Model file for the job. Use its own axes, mm. Give positions to 0.01 mm unless a question says otherwise; leave off trailing zeros. Loops run counter-clockwise (first coordinate to the right, second up) from the corner with the lowest first, then second, coordinate; pieces in that order, holes last. Notation, with made-up numbers: M 66.25,68 L 86.25,68 A29 cw 86.25,98 Z; hole C -22,42.25 d11. An arc over 180 degrees is marked long. Answer in a Markdown table with one row per item.
```python
from build123d import *

# Parameters (mm, degrees)
SKETCH1_R           = 2.875
SKETCH1_R_2         = 7
BOSS_EXTRUDE1_DEPTH = 24.5875
SKETCH4_W           = 66.272407177
SKETCH4_H           = 27.800260981
CUT_EXTRUDE2_DEPTH  = 20
FILLET3_R           = 10
FILLET4_R           = 10
BOSS_EXTRUDE3_START = -1.5875
BOSS_EXTRUDE3_DEPTH = 1.5875
SKETCH7_R           = 7
CUT_EXTRUDE3_DEPTH  = 1.5875
CUT_EXTRUDE4_START  = -10
SKETCH8_R           = 3
SKETCH8_R_2         = 18.9
SKETCH8_R_3         = 2.875
SKETCH8_R_4         = 7
CUT_EXTRUDE4_DEPTH  = 10
SKETCH9_W           = 229.1070397
SKETCH9_H           = 361.266964835
SKETCH9_R           = 1.388229101
SKETCH9_R_2         = 1.483383261
SKETCH9_R_3         = 1.314910669
SKETCH9_R_4         = 1.248623853
SKETCH9_R_5         = 1.255629307
SKETCH9_R_6         = 1.53911217
CUT_EXTRUDE5_DEPTH  = 13
SKETCH10_W          = 29.988446547
SKETCH10_H          = 5
SKETCH10_H_2        = 5.75
CUT_EXTRUDE6_DEPTH  = 22
SKETCH11_R          = 5.236653548
CUT_EXTRUDE7_DEPTH  = 10
BOSS_EXTRUDE4_START = -1.59
BOSS_EXTRUDE4_DEPTH = 1.59
SKETCH13_R          = 7
CUT_EXTRUDE8_DEPTH  = 41
SKETCH14_W          = 61.491848917
SKETCH14_H          = 35.587491391
CUT_EXTRUDE9_DEPTH  = 20
FILLET5_R           = 10
SKETCH16_W          = 163.723031551
SKETCH16_H          = 22.872070304
CUT_EXTRUDE11_DEPTH = 35
FILLET6_R           = 10
SKETCH17_R          = 1.53911217
SKETCH17_R_2        = 1.255629307
SKETCH17_R_3        = 1.3
SKETCH17_R_4        = 1.314910669
SKETCH17_R_5        = 1.388229101
SKETCH17_R_6        = 1.5
CUT_EXTRUDE12_DEPTH = 42
CUT_EXTRUDE13_START = -30
SKETCH18_R          = 18.9
CUT_EXTRUDE13_DEPTH = 30


with BuildPart() as part:
    # Sketch1 → Boss-Extrude1 (new body)
    with BuildSketch(Plane(origin=(0, 0, 0), x_dir=(1, 0, 0), z_dir=(0, 1, 0))):
        with BuildLine():
            Line((42.32729629, 228.6), (10.454309325, 228.6))
            Line((10.454309325, 228.6), (0, 135.362739137))
            Line((0, 135.362739137), (0, 0))
            Line((0, 0), (24.327009544, 0))
            Line((24.327009544, 0), (50.8, 0))
            Line((50.8, 0), (50.8, 64.87909603))
            Line((50.8, 64.87909603), (50.8, 87.423477361))
            Line((50.8, 87.423477361), (50.8, 98.200996728))
            ThreePointArc((50.8, 98.200996728), (50.4, 101.000996728), (50.8, 103.800996728))
            Line((50.8, 103.800996728), (50.8, 104.488200565))
            Line((50.8, 104.488200565), (50.8, 120.619222808))
            Line((50.8, 120.619222808), (50.8, 135.362739137))
            Line((50.8, 135.362739137), (42.32729629, 228.6))
        make_face()
        with Locations(Location((24.101759227, 108.78493524, 0), (0, 0, 270))):
            Circle(SKETCH1_R, mode=Mode.SUBTRACT)
        with Locations(Location((29.504213454, 189.557234372, 0), (0, 0, 270))):
            Circle(SKETCH1_R_2, mode=Mode.SUBTRACT)
    extrude(amount=BOSS_EXTRUDE1_DEPTH)

    # Sketch4 → Cut-Extrude2 (cut)
    with BuildSketch(Plane(origin=(0, 0, -228.6), x_dir=(-1, 0, 0), z_dir=(0, 0, -1))):
        with Locations((-28.174690156, -1.980940155)):
            Rectangle(SKETCH4_W, SKETCH4_H)
    extrude(amount=-CUT_EXTRUDE2_DEPTH, mode=Mode.SUBTRACT)

    # Fillet3
    fillet3_edges = [part.edges().sort_by_distance(p)[0] for p in [
        (44.144746445, 5.959595168, -208.6),
    ]]
    fillet(fillet3_edges, radius=FILLET3_R)

    # Fillet4
    fillet4_edges = [part.edges().sort_by_distance(p)[0] for p in [
        (50.8, 12.29375, 0),
        (0, 12.29375, 0),
        (8.211791854, 5.959595168, -208.6),
    ]]
    fillet(fillet4_edges, radius=FILLET4_R)

    # Sketch6 → Boss-Extrude3 (add)
    with BuildSketch(Plane(origin=(0, 24.5875, 0), x_dir=(1, 0, 0), z_dir=(0, 1, 0)).offset(BOSS_EXTRUDE3_START)):
        with BuildLine():
            Line((50.8, 135.362739137), (50.8, 103.800996728))
            ThreePointArc((50.8, 103.800996728), (50.4, 101.000996728), (50.8, 98.200996728))
            Line((50.8, 98.200996728), (50.8, 61.124243317))
            Line((50.8, 61.124243317), (69.258211507, 96.360728536))
            ThreePointArc((69.258211507, 96.360728536), (70.393157133, 101.370875786), (68.890940865, 106.283413148))
            Line((68.890940865, 106.283413148), (50.8, 135.362739137))
        make_face()
    extrude(amount=BOSS_EXTRUDE3_DEPTH)

    # Sketch7 → Cut-Extrude3 (cut)
    with BuildSketch(Plane(origin=(0, 24.5875, 0), x_dir=(1, 0, 0), z_dir=(0, 1, 0))):
        with Locations(Location((60.4, 101.000996728, 0), (0, 0, 270))):
            Circle(SKETCH7_R)
    extrude(amount=-CUT_EXTRUDE3_DEPTH, mode=Mode.SUBTRACT)

    # Sketch8 → Cut-Extrude4 (cut)
    with BuildSketch(Plane(origin=(0, 24.5875, 0), x_dir=(1, 0, 0), z_dir=(0, 1, 0)).offset(CUT_EXTRUDE4_START)):
        with BuildLine():
            Line((10.454309325, 228.6), (0, 135.362739137))
            Line((0, 135.362739137), (0, 10))
            ThreePointArc((0, 10), (2.928932188, 2.928932188), (10, 0))
            Line((10, 0), (40.8, 0))
            ThreePointArc((40.8, 0), (47.871067812, 2.928932188), (50.8, 10))
            Line((50.8, 10), (50.8, 61.124243317))
            Line((50.8, 61.124243317), (69.258211507, 96.360728536))
            ThreePointArc((69.258211507, 96.360728536), (70.393157133, 101.370875786), (68.890940865, 106.283413148))
            Line((68.890940865, 106.283413148), (50.8, 135.362739137))
            Line((50.8, 135.362739137), (42.32729629, 228.6))
            Line((42.32729629, 228.6), (10.454309325, 228.6))
        make_face()
        with Locations(Location((9.492033273, 118.909935242, 0), (0, 0, 270))):
            Circle(SKETCH8_R, mode=Mode.SUBTRACT)
        with Locations(Location((24.583834565, 64.593886665, 0), (0, 0, 270))):
            Circle(SKETCH8_R_2, mode=Mode.SUBTRACT)
        with Locations(Location((24.101759227, 108.78493524, 0), (0, 0, 270))):
            Circle(SKETCH8_R_3, mode=Mode.SUBTRACT)
        with Locations((60.4, 101.000996728)):
            Circle(SKETCH8_R_4, mode=Mode.SUBTRACT)
        with Locations(Location((29.504213454, 189.557234372, 0), (0, 0, 270))):
            Circle(SKETCH8_R_4, mode=Mode.SUBTRACT)
    extrude(amount=CUT_EXTRUDE4_DEPTH, mode=Mode.SUBTRACT)

    # Sketch9 → Cut-Extrude5 (cut)
    with BuildSketch(Plane.XZ):
        with Locations((19.903204009, -125.752229467)):
            Rectangle(SKETCH9_W, SKETCH9_H)
        with Locations(Location((6.335590122, -44.288799513, 0), (0, 0, 270))):
            Circle(SKETCH9_R, mode=Mode.SUBTRACT)
        with Locations(Location((43.447673368, -42.868436544, 0), (0, 0, 270))):
            Circle(SKETCH9_R_2, mode=Mode.SUBTRACT)
        with Locations(Location((4.659546827, -82.793173401, 0), (0, 0, 270))):
            Circle(SKETCH9_R_3, mode=Mode.SUBTRACT)
        with Locations(Location((48.400988852, -71.551011715, 0), (0, 0, 270))):
            Circle(SKETCH9_R_4, mode=Mode.SUBTRACT)
        with Locations(Location((5.88467603, -135.103145298, 0), (0, 0, 270))):
            Circle(SKETCH9_R_5, mode=Mode.SUBTRACT)
        with Locations(Location((45.747747887, -129.863467374, 0), (0, 0, 270))):
            Circle(SKETCH9_R_6, mode=Mode.SUBTRACT)
    extrude(amount=-CUT_EXTRUDE5_DEPTH, mode=Mode.SUBTRACT)

    # Sketch10 → Cut-Extrude6 (cut)
    with BuildSketch(Plane(origin=(0, 24.5875, 0), x_dir=(1, 0, 0), z_dir=(0, 1, 0))):
        with Locations((23.779803557, 122.41493524)):
            Rectangle(SKETCH10_W, SKETCH10_H)
        with Locations((23.779803557, 108.78493524)):
            Rectangle(SKETCH10_W, SKETCH10_H_2)
        with Locations((23.779803557, 95.528937895)):
            Rectangle(SKETCH10_W, SKETCH10_H)
    extrude(amount=-CUT_EXTRUDE6_DEPTH, mode=Mode.SUBTRACT)

    # Sketch11 → Cut-Extrude7 (cut)
    with BuildSketch(Plane(origin=(0, 24.5875, 0), x_dir=(1, 0, 0), z_dir=(0, 1, 0))):
        with Locations((8.535526315, 118.29502971)):
            Circle(SKETCH11_R)
    extrude(amount=-CUT_EXTRUDE7_DEPTH, mode=Mode.SUBTRACT)

    # Sketch12 → Boss-Extrude4 (add)
    with BuildSketch(Plane(origin=(0, 14.5875, 0), x_dir=(1, 0, 0), z_dir=(0, 1, 0)).offset(BOSS_EXTRUDE4_START)):
        with BuildLine():
            Line((68.287536191, 107.148091395), (50.8, 133.900488173))
            Line((50.8, 133.900488173), (50.8, 103.800996728))
            ThreePointArc((50.8, 103.800996728), (58.520134646, 110.822712782), (68.287536191, 107.148091395))
        make_face()
        with BuildLine():
            Line((69.19540964, 105.759228466), (68.287536191, 107.148091395))
            ThreePointArc((68.287536191, 107.148091395), (58.520134646, 110.822712782), (50.8, 103.800996728))
            ThreePointArc((50.8, 103.800996728), (50.4, 101.000996728), (50.8, 98.200996728))
            ThreePointArc((50.8, 98.200996728), (59.211240578, 91.07190558), (69.067690563, 96.013899345))
            ThreePointArc((69.067690563, 96.013899345), (70.061182785, 98.419999404), (70.4, 101.000996728))
            ThreePointArc((70.4, 101.000996728), (70.094175994, 103.455167016), (69.19540964, 105.759228466))
        make_face()
        with BuildLine():
            ThreePointArc((69.067690563, 96.013899345), (59.211240578, 91.07190558), (50.8, 98.200996728))
            Line((50.8, 98.200996728), (50.8, 64.264230765))
            Line((50.8, 64.264230765), (69.067690563, 96.013899345))
        make_face()
    extrude(amount=BOSS_EXTRUDE4_DEPTH)

    # Sketch13 → Cut-Extrude8 (cut)
    with BuildSketch(Plane(origin=(0, 14.5875, 0), x_dir=(1, 0, 0), z_dir=(0, 1, 0))):
        with Locations(Location((60.4, 101.000996728, 0), (0, 0, 270))):
            Circle(SKETCH13_R)
    extrude(amount=-CUT_EXTRUDE8_DEPTH, mode=Mode.SUBTRACT)

    # Sketch14 → Cut-Extrude9 (cut)
    with BuildSketch(Plane(origin=(0, 0, -228.6), x_dir=(-1, 0, 0), z_dir=(0, 0, -1))):
        with Locations((-33.296946078, 21.381494753)):
            Rectangle(SKETCH14_W, SKETCH14_H)
    extrude(amount=-CUT_EXTRUDE9_DEPTH, mode=Mode.SUBTRACT)

    # Fillet5
    fillet5_edges = [part.edges().sort_by_distance(p)[0] for p in [
        (44.144746445, 13.79375, -208.6),
        (8.211791854, 13.79375, -208.6),
    ]]
    fillet(fillet5_edges, radius=FILLET5_R)

    # Sketch16 → Cut-Extrude11 (cut)
    with BuildSketch(Plane.XY):
        with Locations((6.935844153, 9.456999915)):
            Rectangle(SKETCH16_W, SKETCH16_H)
    extrude(amount=-CUT_EXTRUDE11_DEPTH, mode=Mode.SUBTRACT)

    # Fillet6
    fillet6_edges = [part.edges().sort_by_distance(p)[0] for p in [
        (0, 13.79375, -35),
        (50.8, 13.79375, -35),
    ]]
    fillet(fillet6_edges, radius=FILLET6_R)

    # Sketch17 → Cut-Extrude12 (cut)
    with BuildSketch(Plane.XZ):
        with Locations(Location((45.747747887, -129.863467374, 0), (0, 0, 270))):
            Circle(SKETCH17_R)
        with Locations(Location((5.88467603, -135.103145298, 0), (0, 0, 270))):
            Circle(SKETCH17_R_2)
        with Locations(Location((48.400988852, -71.551011715, 0), (0, 0, 270))):
            Circle(SKETCH17_R_3)
        with Locations(Location((4.659546827, -82.793173401, 0), (0, 0, 270))):
            Circle(SKETCH17_R_4)
        with Locations(Location((6.335590122, -44.288799513, 0), (0, 0, 270))):
            Circle(SKETCH17_R_5)
        with Locations(Location((43.447673368, -42.868436544, 0), (0, 0, 270))):
            Circle(SKETCH17_R_6)
    extrude(amount=-CUT_EXTRUDE12_DEPTH, mode=Mode.SUBTRACT)

    # Sketch18 → Cut-Extrude13 (cut)
    with BuildSketch(Plane(origin=(0, 24.5875, 0), x_dir=(1, 0, 0), z_dir=(0, 1, 0)).offset(CUT_EXTRUDE13_START)):
        with Locations(Location((24.583834565, 64.593886665, 0), (0, 0, 270))):
            Circle(SKETCH18_R)
    extrude(amount=CUT_EXTRUDE13_DEPTH, mode=Mode.SUBTRACT)


solid = part.part
```
Q1. Mould opens along X. For faces 1 (the face through (3.01, 13.78, -37.85)), 2 (the face through (45.815, 13.783, -128.326)), 3 (the face through (51, 12.998, -100)) say: released by +X, released by -X, zero draft, split by the parting line, or undercut.
Reported:
| item | result |
|---|---|
| face 1 | released by -X |
| face 2 | undercut |
| face 3 | zero draft |
Q2. Saw through at C-C (y = 14.1). Give the number of separate pieces and of enclosed holes in the cut face, and give its area (3 significant figures).
Reported:
| item | result |
|---|---|
| separate pieces | 1 |
| enclosed holes | 12 |
| area | 6,990 mm² |
Q3. Saw through at A-A (x = 19). Give the cut face in (y, z).
Reported:
| item | result |
|---|---|
| outline | M 13,-208.6 L 14.59,-208.6 L 14.59,-124.91 L 13,-124.91 Z; M 13,-119.91 L 14.59,-119.91 L 14.59,-111.66 L 13,-111.66 Z; M 13,-105.91 L 14.59,-105.91 L 14.59,-98.03 L 13,-98.03 Z; M 13,-93.03 L 14.59,-93.03 L 14.59,-82.65 L 13,-82.65 Z; M 13,-46.54 L 14.59,-46.54 L 14.59,-35 L 13,-35 Z |
Q4. Drop a flat-ended pin along its axis: pin 1 (0.7 mm diameter, centred on y = 14, z = -135, fed in from +X). Give the stop position or say it passes through.
Reported:
| item | result |
|---|---|
| pin 1 | x = 50.8 |
Q5. Probe probe 1 along Z at (x, y) = (22, 13.4); probe 2 along Z at (x, y) = (19.5, 13.5); probe 3 along X at (y, z) = (13.8, -71). List the from-to ranges inside material, lowest first.
Reported:
| item | result |
|---|---|
| probe 1 | -208.6 to -124.91, -119.91 to -111.66, -105.91 to -98.03, -93.03 to -83.32, -45.87 to -35 |
| probe 2 | -208.6 to -124.91, -119.91 to -111.66, -105.91 to -98.03, -93.03 to -82.8, -46.39 to -35 |
| probe 3 | 0 to 6.8, 42.37 to 47.22, 49.58 to 54.68 |
Q6. Saw through at D-D (z = -172). Give the cut face in (x, y), and give its area (3 significant figures).
Reported:
| item | result |
|---|---|
| outline | M 4.11,13 L 47.47,13 L 47.47,14.59 L 4.11,14.59 Z |
| area | 68.8 mm² |
Q7. Saw through at B-B (x = 60.4). Give the cut face in (y, z), and give its area (3 significant figures).
Reported:
| item | result |
|---|---|
| outline | M 13,-119.21 L 14.59,-119.21 L 14.59,-108 L 13,-108 Z; M 13,-94 L 14.59,-94 L 14.59,-80.95 L 13,-80.95 Z |
| area | 38.6 mm² |
